from build123d import *

# Parameters (mm, degrees)
BOSS_EXTRUDE1_DEPTH = 10
CUT_EXTRUDE1_DEPTH  = 11
FILLET1_R           = 5
SKETCH3_W           = 40
SKETCH3_H           = 20
BOSS_EXTRUDE2_DEPTH = 5
SKETCH4_R           = 1.75
CUT_EXTRUDE2_DEPTH  = 16
FILLET2_R           = 4


with BuildPart() as part:
    # Sketch1 → Boss-Extrude1 (new body, symmetric)
    with BuildSketch(Plane(origin=(0, 0, 0), x_dir=(0, 0, -1), z_dir=(1, 0, 0))):
        Polygon((0, 0), (0, -35), (-10, -35), (-10, 10), align=None)
    extrude(amount=BOSS_EXTRUDE1_DEPTH, both=True)

    # Sketch2 → Cut-Extrude1 (cut, through all)
    with BuildSketch(Plane.XY.offset(10)):
        with BuildLine():
            Line((1.75, -5), (1.75, -30))
            ThreePointArc((1.75, -30), (0, -31.75), (-1.75, -30))
            Line((-1.75, -30), (-1.75, -5))
            ThreePointArc((-1.75, -5), (0, -3.25), (1.75, -5))
        make_face()
    extrude(amount=-CUT_EXTRUDE1_DEPTH, mode=Mode.SUBTRACT)

    # Fillet1
    fillet1_edges = [part.edges().sort_by_distance(p)[0] for p in [
        (10, -35, 5),
        (-10, -35, 5),
    ]]
    fillet(fillet1_edges, radius=FILLET1_R)

    # Sketch3 → Boss-Extrude2 (add)
    with BuildSketch(Plane(origin=(0, 0, 0), x_dir=(1, 0, 0), z_dir=(0, 0.707106781, -0.707106781))):
        with Locations((0, -10)):
            Rectangle(SKETCH3_W, SKETCH3_H)
    extrude(amount=BOSS_EXTRUDE2_DEPTH)

    # Sketch4 → Cut-Extrude2 (cut, through all)
    with BuildSketch(Plane(origin=(0, 0, 0), x_dir=(1, 0, 0), z_dir=(0, -0.707106781, 0.707106781))):
        with Locations((-15, 10)):
            Circle(SKETCH4_R)
        with Locations((15, 10)):
            Circle(SKETCH4_R)
    extrude(amount=-CUT_EXTRUDE2_DEPTH, mode=Mode.SUBTRACT)

    # Fillet2
    fillet2_edges = [part.edges().sort_by_distance(p)[0] for p in [
        (-20, 1.767766953, -1.767766953),
        (-20, 15.909902577, 12.374368671),
        (20, 15.909902577, 12.374368671),
        (20, 1.767766953, -1.767766953),
    ]]
    fillet(fillet2_edges, radius=FILLET2_R)


solid = part.part
Geometry: final body of the model. Coordinates: model frame, mm. A direction names the side the tool comes from. Give positions to 0.01 mm unless a question says otherwise; leave off trailing zeros. Write each loop counter-clockwise with the first axis right and the second up, starting at its lowest first coordinate (ties: lowest second). Pieces come first, ordered by that corner, then holes.
(1) Cut plane D-D, the plane y = -1.5. Return loops of the section in (x, z), then the cut area to 3 significant figures.
(2) First-contact query: P1, Ø10, axis at x = 3.5, y = 4, coming from the +Z side; P2, Ø8, axis at y = -12, z = 6.5, coming from the +X side; P3, Ø5, axis at y = -12.5, z = -1.5, coming from the -X side; P4, Ø6, axis at x = -6.5, z = 7, coming from the -Y side. Flat tips, straight axial feed; report the tip coordinate or a pass-through.
(3) Access query for faces 1 (the flat face through (-0.28, 10.11, 10.11)), 2 (the flat face through (-1.75, -18, 5)), 3 (the flat face through (-2, -13, 10)), 4 (the flat face through (-0.224, 15.885, 12.399)), 5 (the cylindrical face through (-18.86, 2.64, -0.94)). Directions: +Z, -Z, +X, -X, +Y, -Y. A direction counts if a zero-diameter tool reaches every point of the face in a straight line with its end or side. Return the directions, or none.
(4) Cut plane A-A, the plane y = -7. Return loops of the section in (x, z).
(5) Ray query, line 1 (X direction, y = -7.5, z = 4.75); line 2 (Z direction, x = -8, y = -20.5); line 3 (Y direction, x = -6, z = 11.5). Return the intervals inside material, ascending.
(6) Cut plane B-B, the plane x = 0. Return loops of the section in (y, z), then the cut area to 3 significant figures.
(7) Mould query, pull axis X, two halves, no side actions, for faces 6 (the flat face through (-0.28, 10.51, 3.44)), 7 (the cylindrical face through (16.67, 9.19, 5.7)), 8 (the flat face through (-20, 9, 5)). Classes: released by +X, released by -X, zero draft, split by the parting line, or undercut.
(8) Cut plane C-C, the plane x = -9. Return loops of the section in (y, z), then the cut area to 3 significant figures.
Values follow:
1. outline: (-10, 0) - (10, 0) - (10, 10) - (-10, 10) - close
1. area: 200 mm2
2. P1: stops at z = 10
2. P2: stops at x = 10
2. P3: stops at x = -10
2. P4: stops at y = -35
3. face 1: +Z, -Y
3. face 2: +Z, -Z
3. face 3: +Z, +X, -X, -Y
3. face 4: +Z, +X, -X, +Y
3. face 5: -Z, -X, -Y
4. outline: (-10, 0) - (-1.75, 0) - (-1.75, 10) - (-10, 10) - close; (1.75, 0) - (10, 0) - (10, 10) - (1.75, 10) - close
5. line 1: x = -10 to -1.75, 1.75 to 10
5. line 2: z = 0 to 10
5. line 3: y = 11.5 to 16.78
6. outline: (-35, 0) - (-31.75, 0) - (-31.75, 10) - (-35, 10) - close; (-3.25, 0) - (0, 0) - (3.54, -3.54) - (17.68, 10.61) - (14.14, 14.14) - (10, 10) - (-3.25, 10) - close
6. area: 215 mm2
7. face 6: zero draft
7. face 7: undercut
7. face 8: released by -X
8. outline: (-33, 0) - (0, 0) - (3.54, -3.54) - (17.68, 10.61) - (14.14, 14.14) - (10, 10) - (-33, 10) - close
8. area: 480 mm2
